For this review, use the dimensioned drawing (mm, ordinates from the lowest corner) and the shaded views. Give positions to 0.01 mm unless a question says otherwise; leave off trailing zeros. Write each loop counter-clockwise with the first axis right and the second up, starting at its lowest first coordinate (ties: lowest second). Pieces come first, ordered by that corner, then holes.
1) We need section C-C on x = 4. Give the boundary of the cut face in (y, z), and give its area (3 significant figures).
2) We need section A-A on z = 1. Give the boundary of the cut face in (x, y), and give its area (3 significant figures).
3) We need section B-B on y = 17. Give the boundary of the cut face in (x, z).
4) Wall thickness on line 1 along Y through (x, z) = (4, 0.9); line 2 along Z through (x, y) = (6.75, 10.25); line 3 along X through (y, z) = (8, 1.3): over which ranges is each line inside the solid? List them lowest first.
5) For P1, Ø0.9, axis at x = 3.5, z = 1.5, coming from the -Y side; P2, Ø0.7, axis at x = 3.5, z = 1.5, coming from the +Y side; P3, Ø0.7, axis at x = 4.5, z = 1, coming from the +Y side, all flat-tipped, find the tip position at first contact; note any pin that passes through.
6) We need section D-D on x = 2.5. Give the boundary of the cut face in (y, z).
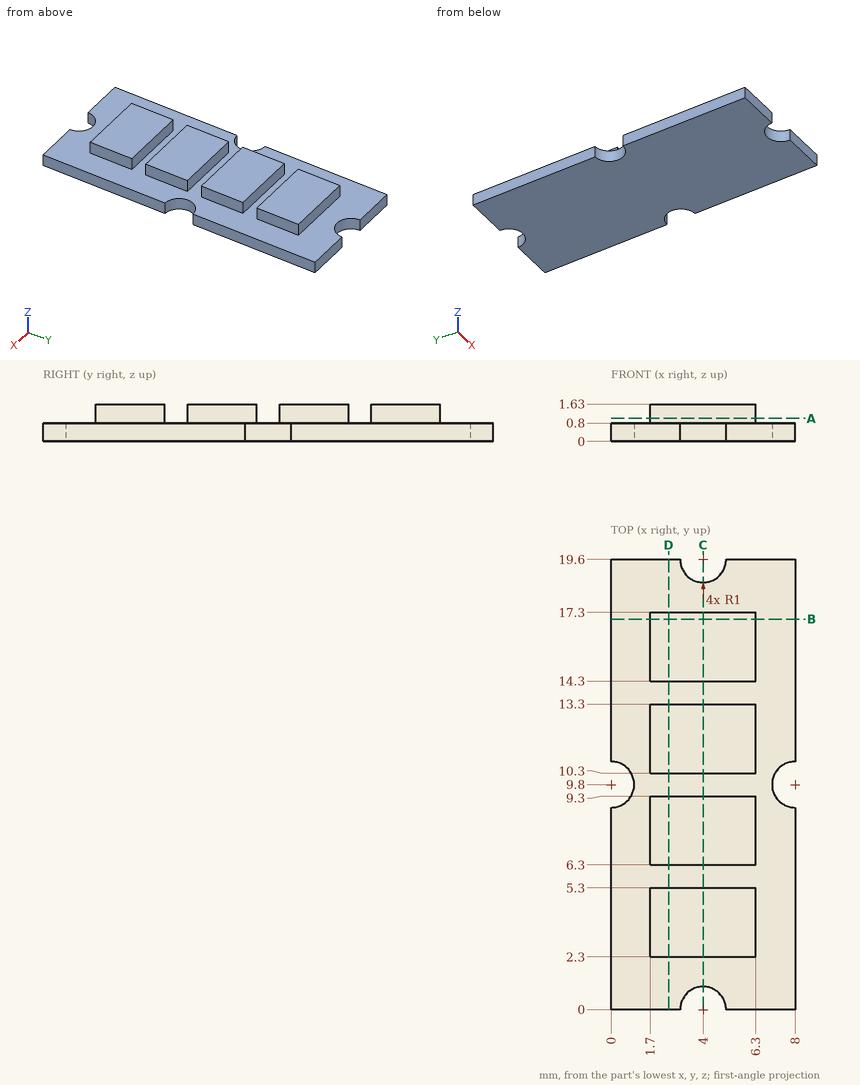
Results list:
1. outline: (1, 0) - (18.6, 0) - (18.6, 0.8) - (17.3, 0.8) - (17.3, 1.63) - (14.3, 1.63) - (14.3, 0.8) - (13.3, 0.8) - (13.3, 1.63) - (10.3, 1.63) - (10.3, 0.8) - (9.3, 0.8) - (9.3, 1.63) - (6.3, 1.63) - (6.3, 0.8) - (5.3, 0.8) - (5.3, 1.63) - (2.3, 1.63) - (2.3, 0.8) - (1, 0.8) - close
1. area: 24.0 mm2
2. outline: (1.7, 2.3) - (6.3, 2.3) - (6.3, 5.3) - (1.7, 5.3) - close; (1.7, 6.3) - (6.3, 6.3) - (6.3, 9.3) - (1.7, 9.3) - close; (1.7, 10.3) - (6.3, 10.3) - (6.3, 13.3) - (1.7, 13.3) - close; (1.7, 14.3) - (6.3, 14.3) - (6.3, 17.3) - (1.7, 17.3) - close
2. area: 55.2 mm2
3. outline: (0, 0) - (8, 0) - (8, 0.8) - (6.3, 0.8) - (6.3, 1.63) - (1.7, 1.63) - (1.7, 0.8) - (0, 0.8) - close
4. line 1: y = 2.3 to 5.3, 6.3 to 9.3, 10.3 to 13.3, 14.3 to 17.3
4. line 2: z = 0 to 0.8
4. line 3: x = 1.7 to 6.3
5. P1: stops at y = 2.3
5. P2: stops at y = 17.3
5. P3: stops at y = 18.98
6. outline: (0, 0) - (19.6, 0) - (19.6, 0.8) - (17.3, 0.8) - (17.3, 1.63) - (14.3, 1.63) - (14.3, 0.8) - (13.3, 0.8) - (13.3, 1.63) - (10.3, 1.63) - (10.3, 0.8) - (9.3, 0.8) - (9.3, 1.63) - (6.3, 1.63) - (6.3, 0.8) - (5.3, 0.8) - (5.3, 1.63) - (2.3, 1.63) - (2.3, 0.8) - (0, 0.8) - close
